from build123d import *

# Parameters (mm, degrees)
SKETCH1_W           = 20
SKETCH1_H           = 23
BOSS_EXTRUDE1_DEPTH = 3
SKETCH2_W           = 20
SKETCH2_H           = 3
BOSS_EXTRUDE2_DEPTH = 20
SKETCH3_R           = 5
BOSS_EXTRUDE3_DEPTH = 25
SKETCH4_R           = 3
CUT_EXTRUDE1_DEPTH  = 25
SKETCH5_W           = 23
SKETCH5_H           = 3
BOSS_EXTRUDE4_DEPTH = 87
SKETCH6_R           = 2.5
CUT_EXTRUDE2_DEPTH  = 3


with BuildPart() as part:
    # Sketch1 → Boss-Extrude1 (new body)
    with BuildSketch(Plane.XY):
        with Locations((10, -11.5)):
            Rectangle(SKETCH1_W, SKETCH1_H)
    extrude(amount=BOSS_EXTRUDE1_DEPTH)

    # Sketch2 → Boss-Extrude2 (add)
    with BuildSketch(Plane.XY.offset(3)):
        with Locations((10, -1.5)):
            Rectangle(SKETCH2_W, SKETCH2_H)
    extrude(amount=BOSS_EXTRUDE2_DEPTH)

    # Sketch3 → Boss-Extrude3 (add)
    with BuildSketch(Plane(origin=(0, 0, 0), x_dir=(-1, 0, 0), z_dir=(0, 0, -1))):
        with Locations((-10, -13)):
            Circle(SKETCH3_R)
    extrude(amount=BOSS_EXTRUDE3_DEPTH)

    # Sketch4 → Cut-Extrude1 (cut)
    with BuildSketch(Plane(origin=(0, 0, -25), x_dir=(-1, 0, 0), z_dir=(0, 0, -1))):
        with Locations((-10, -13)):
            Circle(SKETCH4_R)
    extrude(amount=-CUT_EXTRUDE1_DEPTH, mode=Mode.SUBTRACT)

    # Sketch5 → Boss-Extrude4 (add)
    with BuildSketch(Plane.ZY):
        with Locations((11.5, -1.5)):
            Rectangle(SKETCH5_W, SKETCH5_H)
    extrude(amount=BOSS_EXTRUDE4_DEPTH)

    # Sketch6 → Cut-Extrude2 (cut)
    with BuildSketch(Plane(origin=(0, 0, 0), x_dir=(1, 0, 0), z_dir=(0, 1, 0))):
        with Locations(Location((-82.9, -11.5, 0), (0, 0, 270))):
            Circle(SKETCH6_R)
    extrude(amount=-CUT_EXTRUDE2_DEPTH, mode=Mode.SUBTRACT)


solid = part.part
Verification items for the finished model (mm, model axes). A direction names the side the tool comes from. Give positions to 0.01 mm unless a question says otherwise; leave off trailing zeros. Order: outer loops, then holes, each group sorted by start corner. A loop starts at its lowest first (then second) coordinate and runs counter-clockwise, first axis right, second up. Notation, with made-up numbers: M 64.25,89.25 L 102.25,89.25 A22 cw 102.25,111.25 Z; hole C 37,63 d10. An arc over 180 degrees is marked long. Use one line per item in the form item = value. Start each with the question number.
Q1. Go/stop test with flat-tipped pins: pin 1 Ø10 at (x, z) = (-7.5, -3) entering from +Y; pin 2 Ø2.5 at (y, z) = (-13, 2) entering from -X; pin 3 Ø10 at (y, z) = (-8, -12.5) entering from +X; pin 4 Ø5.5 at (x, y) = (10, -13) entering from -Z. Record where each tip stops, or that it passes through.
Q2. Access from +Z, -Z, +X, -X, +Y, -Y to the whole of each face (thin tool, end or side, straight path). Record for faces 1 (the flat face through (10, -13, 0)), 2 (the flat face through (10, -13, 3)), 3 (the flat face through (0, -13, 1)).
Q3. Scan lines: line 1 along X through (y, z) = (-2.3, 11.5); line 2 along Y through (x, z) = (-28, 16); line 3 along Z through (x, y) = (-77, -1). Record each from-to range of solid material in increasing order. Write a range as [from, to].
Q4. Section check D-D (x = 10). Enter the section's corners in (y, z).
Q5. Mould release check, pull along X, two halves, no side actions. Record for faces 4 (the cylindrical face through (5.23, -11.5, -12.32)), 5 (the cylindrical face through (12.4, -14.8, -12.7)), 6 (the flat face through (20, -7, 2)): +X half, -X half, draft (parallel to the pull), parting line (faces both ways), or undercut.
Q6. Section check A-A (z = 11.5). Enter the section's corners in (x, y), then the cut area to 3 significant figures.
Q7. Section check C-C (y = -17). Enter the section's corners in (x, z).
Q8. Section check B-B (x = -82.9). Enter the section's corners in (y, z), then the cut area to 3 significant figures.
Evaluation:
q1.pin_1 = 0
q1.pin_2 = 0
q1.pin_3 = 15
q1.pin_4 = 0
q2.face_1 = -Z
q2.face_2 = +Z, +X, -X, -Y
q2.face_3 = +Z, -Z, -X, -Y
q3.line_1 = [-87, -85.4], [-80.4, 20]
q3.line_2 = [-3, 0]
q3.line_3 = [0, 23]
q4.outline = M -23,0 L -18,0 L -18,-25 L -16,-25 L -16,0 L -10,0 L -10,-25 L -8,-25 L -8,0 L 0,0 L 0,23 L -3,23 L -3,3 L -23,3 Z
q5.face_4 = parting line
q5.face_5 = undercut
q5.face_6 = +X half
q6.outline = M -87,-3 L -85.4,-3 L -85.4,0 L -87,0 Z; M -80.4,-3 L 20,-3 L 20,0 L -80.4,0 Z
q6.area = 306 mm2
q7.outline = M 0,0 L 7,0 L 7,-25 L 13,-25 L 13,0 L 20,0 L 20,3 L 0,3 Z
q8.outline = M -3,0 L 0,0 L 0,9 L -3,9 Z; M -3,14 L 0,14 L 0,23 L -3,23 Z
q8.area = 54.0 mm2
